Geometry check sheet. Reference: the model listing, model coordinates, mm. Coordinates: 2 decimals unless noted, no trailing zeros. Order: outer loops, then holes, each group sorted by start corner. A loop starts at its lowest first (then second) coordinate and runs counter-clockwise, first axis right, second up. Notation, with made-up numbers: (19.5, -19) -> (46.5, -19) arc R13 ccw to (46.5, 5) -> close; hole circle Ø1 at (-12, 20). An arc over 180 degrees is marked (long way). Answer in a Markdown table with one row per item. Add a question column.
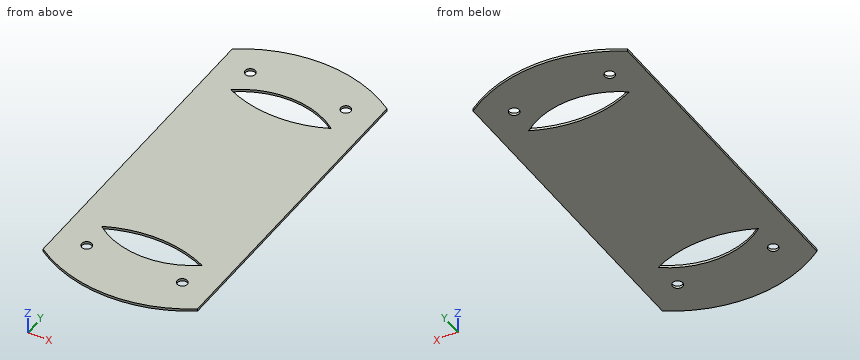
Autodesk Inventor part; units mm, degrees
ref_plane "YZ Plane" through (0, 0, 0) normal (1, 0, 0) x (0, 1, 0)
ref_plane "XZ Plane" through (0, 0, 0) normal (0, 1, 0) x (-1, 0, 0)
ref_plane "XY Plane" through (0, 0, 0) normal (0, 0, 1) x (1, 0, 0)
sketch "Szkic1" plane through (0, 0, 0) normal (0, 0, 1) x (1, 0, 0)
  circle A0 centre (-19, 53.736463) radius 2
  line L0 (0, -102.826606) -> (0, 109.459635)
  circle A1 centre (51.489502, -156.180896) radius 2
  circle A2 centre (-19, -53.736463) radius 2
  circle A3 centre (19, -53.736463) radius 2
  spline S0 degree 3 poles (-19.948357, 42.291714) (-7.484612, 36.499399) (6.838806, 36.499399) (19.884685, 42.334177) knots -2 -2 -2 -2 -1 -1 -1 -1
  spline S1 degree 3 poles (19.884685, 42.334177) (18.683547, 43.134298) (16.314211, 44.578944) (13.440795, 46.011363) (10.633281, 47.178527) (8.438356, 47.906787) (5.748573, 48.576507) (3.633449, 48.926153) (1.014806, 49.141741) (-1.070138, 49.1397) (-3.689231, 48.918937) (-5.805048, 48.565032) (-8.496008, 47.889736) (-10.692066, 47.156791) (-13.501106, 45.983476) (-16.376096, 44.544624) (-18.746641, 43.094581) (-19.948357, 42.291714) knots -1.92878405 -1.92878405 -1.92878405 -1.92878405 -1.85742515 -1.78606626 -1.75038681 -1.67902792 -1.64334847 -1.57198957 -1.53631013 -1.46495123 -1.42927178 -1.35791289 -1.32223344 -1.25087454 -1.2151951 -1.1438362 -1.0724773 -1.0724773 -1.0724773 -1.0724773
  spline S2 degree 3 poles (-19.948357, -42.291714) (-7.484612, -36.499399) (6.838806, -36.499399) (19.884685, -42.334177) (19.887771, -42.335557) (19.890857, -42.336938) (19.893943, -42.338318) knots -2 -2 -2 -2 -1 -1 -1 -0.99976344 -0.99976344 -0.99976344 -0.99976344
  arc A4 (10.816477, 63.441394) -> (10.816477, 63.441394) centre (0.029646, 15.697095) ccw
  line L1 (-30.717431, -63.122795) -> (-30.717431, 61.299929)
  line L2 (30.776723, 61.29993) -> (30.717431, -63.122795)
  arc A5 (46.460279, 45.179229) -> (46.388819, 45.291469) centre (0.029646, 15.697095) ccw
  arc A6 (30.776723, 61.29993) -> (-30.717431, 61.299929) centre (0.029646, 15.697095) ccw
  arc A7 (-30.717431, -63.122795) -> (30.717431, -63.122795) centre (0, -17.5) ccw
  spline S3 degree 3 poles (19.884685, -42.334177) (18.683547, -43.134298) (16.314211, -44.578944) (13.440795, -46.011363) (10.633281, -47.178527) (8.438356, -47.906787) (5.748573, -48.576507) (3.633449, -48.926153) (1.014806, -49.141741) (-1.070138, -49.1397) (-3.689231, -48.918937) (-5.805048, -48.565032) (-8.496008, -47.889736) (-10.692066, -47.156791) (-13.501106, -45.983476) (-16.376096, -44.544624) (-18.746641, -43.094581) (-19.948357, -42.291714) knots -1.92878405 -1.92878405 -1.92878405 -1.92878405 -1.85742515 -1.78606626 -1.75038681 -1.67902792 -1.64334847 -1.57198957 -1.53631013 -1.46495123 -1.42927178 -1.35791289 -1.32223344 -1.25087454 -1.2151951 -1.1438362 -1.0724773 -1.0724773 -1.0724773 -1.0724773
  arc A8 (-19.985617, 42.471752) -> (20.021799, 42.489012) centre (0, 84.415359) ccw
  arc A9 (20.021799, 42.489012) -> (-19.985617, 42.471752) centre (0.029646, 15.697095) ccw
  arc A10 (31.190436, 27.800736) -> (30.76126, 28.852355) centre (0.029646, 15.697095) ccw
  line L3 (-47.966946, 0) -> (72.77966, 0)
  arc A11 (20.021799, -42.489012) -> (-19.985617, -42.471752) centre (0, -84.415359) ccw
  arc A12 (-19.985617, -42.471752) -> (20.021799, -42.489012) centre (0.029646, -15.697095) ccw
  line L4 (0, -211.709002) -> (0, 162.987741)
  circle A13 centre (19, 53.736463) radius 2
  point P0 (0, 0)
  point P1 (0.029639, 15.697104)
  dimension "d0" = 4
sketch "Szkic1 outline for Wyciągnięcie proste1" plane through (0, 0, 0) normal (0, 0, 1) x (1, 0, 0)
  line L0 (-30.717431, -63.122795) -> (-30.717431, 61.299929)
  arc A0 (30.717431, -63.122795) -> (-30.717431, -63.122795) centre (0, -17.5) cw
  arc A1 (-30.717431, 61.299929) -> (30.776723, 61.29993) centre (0.029646, 15.697095) cw
  line L1 (30.776723, 61.29993) -> (30.717431, -63.122795)
  circle A2 centre (-19, -53.736463) radius 2
  arc A3 (20.021799, -42.489012) -> (-19.985617, -42.471752) centre (0, -84.415359) ccw
  arc A4 (-19.985617, -42.471752) -> (20.021799, -42.489012) centre (0.029646, -15.697095) ccw
  circle A5 centre (19, -53.736463) radius 2
  circle A6 centre (-19, 53.736463) radius 2
  arc A7 (-19.985617, 42.471752) -> (20.021799, 42.489012) centre (0.029646, 15.697095) cw
  arc A8 (20.021799, 42.489012) -> (-19.985617, 42.471752) centre (0, 84.415359) cw
  circle A9 centre (19, 53.736463) radius 2
extrude "Wyciągnięcie proste1" add sketch "Szkic1 outline for Wyciągnięcie proste1" along normal blind 1
sketch "Szkic2" plane through (0, 0, 1) normal (0, 0, 1) x (1, 0, 0)
  spline S0 degree 3 poles (19.066093, -42.869125) (17.919263, -43.604012) (15.656614, -44.931314) (12.910224, -46.24893) (10.224207, -47.323895) (8.121883, -47.995773) (5.542498, -48.61482) (3.51191, -48.938928) (0.996255, -49.139822) (-1.007288, -49.139431) (-3.523026, -48.937545) (-5.553743, -48.612623) (-8.133347, -47.992513) (-10.235885, -47.319744) (-12.922191, -46.24361) (-15.668883, -44.924773) (-17.931768, -43.596446) (-19.078711, -42.861037) knots 1.08873831 1.08873831 1.08873831 1.08873831 1.15730288 1.22586745 1.26014974 1.32871431 1.36299659 1.43156116 1.46584345 1.53440802 1.5686903 1.63725487 1.67153715 1.74010172 1.77438401 1.84294858 1.91151315 1.91151315 1.91151315 1.91151315
  spline S1 degree 2 poles (-19.078711, -42.861037) (-0.031622, -36.330707) (19.066093, -42.869125) knots 1.17954056 1.17954056 1.17954056 1.82085643 1.82085643 1.82085643
  point P0 (0, 0)
extrude "Wyciągnięcie proste2" cut sketch "Szkic2" against normal through all
properties part number "plyta_odbiornik"
(1) Go/stop test with a flat-tipped pin: P1, Ø4.5, axis at x = 19, y = 53.74, coming from the +Z side. Record where the tip stops, or that it passes through.
(2) Cross-section at A-A (z = 0.4). Enter the section's corners in (x, y).
(3) Cross-section at B-B (x = -14). Enter the section's corners in (y, z).
(4) Cross-section at C-C (y = -47). Enter the section's corners in (x, z), plus the area to 3 significant figures.
(5) Cross-section at D-D (x = -2). Enter the section's corners in (y, z), plus the area to 3 significant figures.
(6) Scan lines: line 1 along X through (y, z) = (54, 0.9); line 2 along Y through (x, z) = (10, 0.5); line 3 along Y through (x, z) = (7, 0.35). Record each from-to range of solid material in increasing order.
Checks:
| question | item | result |
|---|---|---|
| 1 | P1 | z = 1 |
| 2 | outline | (-30.72, -63.12) arc R55 ccw to (30.72, -63.12) -> (30.78, 61.3) arc R55 ccw to (-30.72, 61.3) -> close; hole circle Ø4 at (-19, -53.74); hole circle Ø4 at (-19, 53.74); hole (-19.99, -42.47) arc R33.43 ccw to (20.02, -42.49) arc R46.46 ccw to start; hole (-19.99, 42.47) arc R46.46 ccw to (20.02, 42.49) arc R33.43 ccw to start; hole circle Ø4 at (19, -53.74); hole circle Ø4 at (19, 53.74) |
| 3 | outline | (-70.69, 0) -> (-46.04, 0) -> (-46.04, 1) -> (-70.69, 1) -> close; (-40.11, 0) -> (40.11, 0) -> (40.11, 1) -> (-40.11, 1) -> close; (46.04, 0) -> (68.88, 0) -> (68.88, 1) -> (46.04, 1) -> close |
| 4 | outline | (-30.72, 0) -> (-11.7, 0) -> (-11.7, 1) -> (-30.72, 1) -> close; (11.76, 0) -> (30.73, 0) -> (30.73, 1) -> (11.76, 1) -> close |
| 4 | area | 38.0 mm² |
| 5 | outline | (-72.46, 0) -> (-49.06, 0) -> (-49.06, 1) -> (-72.46, 1) -> close; (-38, 0) -> (38, 0) -> (38, 1) -> (-38, 1) -> close; (49.06, 0) -> (70.66, 0) -> (70.66, 1) -> (49.06, 1) -> close |
| 5 | area | 121 mm² |
| 6 | line 1 | -30.72 to -20.98, -17.02 to 17.02, 20.98 to 30.77 |
| 6 | line 2 | -71.58 to -47.6, -39.04 to 39.04, 47.6 to 69.79 |
| 6 | line 3 | -72.05 to -48.39, -38.48 to 38.48, 48.39 to 70.25 |
